Autodesk Inventor part; units mm, degrees
ref_plane "YZ Plane" through (0, 0, 0) normal (1, 0, 0) x (0, 1, 0)
ref_plane "XZ Plane" through (0, 0, 0) normal (0, 1, 0) x (-1, 0, 0)
ref_plane "XY Plane" through (0, 0, 0) normal (0, 0, 1) x (1, 0, 0)
sketch "Skizze1" plane through (0, 0, 0) normal (0, 0, 1) x (1, 0, 0)
  line L0 (0, 0) -> (90.4, 0)
  line L1 (90.4, 0) -> (90.4, 80)
  line L2 (90.4, 80) -> (0, 80)
  line L3 (0, 80) -> (0, 0)
  line L4 (2.6, 69.1) -> (87.8, 69.1) construction
  line L5 (87.8, 69.1) -> (87.8, 10.9) construction
  circle A0 centre (2.6, 69.1) radius 1.6
  circle A1 centre (2.6, 10.9) radius 1.6
  circle A2 centre (87.8, 69.1) radius 1.6
  circle A3 centre (87.8, 10.9) radius 1.6
  line L6 (65.2, 69.1) -> (82.75, 69.1) construction
  line L7 (25.2, 69.1) -> (42.75, 69.1) construction
  dimension "d0" = 90.4
  dimension "d1" = 80
  dimension "d5" = 87.8
  dimension "d6" = 3.2
extrude "Extrusion1" add sketch "Skizze1" along normal blind 2
chamfer "Fase1" distance 1.6 angle 45 4 edges at (86.2, 10.9, 2) (1, 10.9, 2) (1, 69.1, 2) (86.2, 69.1, 2)
properties part number "blech_2mm"
The model under review builds one solid part; all positions refer to its coordinate system, in mm. Coordinates: 2 decimals unless noted, no trailing zeros. Write each loop counter-clockwise with the first axis right and the second up, starting at its lowest first coordinate (ties: lowest second). Pieces come first, ordered by that corner, then holes. Notation, with made-up numbers: (59.25, -26) - (102.25, -26) arc R9 cw to (102.25, -11) - close; hole circle Ø4 at (17, -18.5). An arc over 180 degrees is marked (long way). Answer in a Markdown table with one row per item. Add a question column.
Q1. To check wall thickness, follow line 1 along Y through (x, z) = (87.8, 0.1); line 2 along X through (y, z) = (69.1, 0.2); line 3 along X through (y, z) = (11.5, 0.2). State the ranges of each line that lie inside material, in increasing order. Write a range as from..to.
Q2. Clearance check with flat-ended pins moving along their axes: pin 1 (4 mm diameter, centred on x = 87.8, y = 10.9, fed in from +Z); pin 2 (3 mm diameter, centred on x = 87.8, y = 69.1, fed in from +Z); pin 3 (5 mm diameter, centred on x = 2.6, y = 69.1, fed in from +Z). State where each tip first meets the part, or that it passes through.
Q3. Consider section A-A on x = 87.8. Give the boundary of the cut face in (y, z).
Q4. Consider section B-B on y = 10.9. Give the boundary of the cut face in (x, z).
Q5. Draft analysis for pull direction X (two halves, no side actions). For faces 1 (the face through (4.335, 10.181, 0.678)), 2 (the face through (45, 0, 1)), 3 (the face through (0, 41, 1)), state which applies: +X half, -X half, draft (parallel to the pull), parting line (faces both ways), or undercut.
Answers below:
| question | item | result |
|---|---|---|
| 1 | line 1 | 0..9.3, 12.5..67.5, 70.7..80 |
| 1 | line 2 | 0..1, 4.2..86.2, 89.4..90.4 |
| 1 | line 3 | 0..1.12, 4.08..86.32, 89.28..90.4 |
| 2 | pin 1 | z = 0.8 |
| 2 | pin 2 | through |
| 2 | pin 3 | z = 1.3 |
| 3 | outline | (0, 0) - (9.3, 0) - (9.3, 0.4) - (7.7, 2) - (0, 2) - close; (12.5, 0) - (67.5, 0) - (67.5, 0.4) - (65.9, 2) - (14.1, 2) - (12.5, 0.4) - close; (70.7, 0) - (80, 0) - (80, 2) - (72.3, 2) - (70.7, 0.4) - close |
| 4 | outline | (0, 0) - (1, 0) - (1, 0.4) - (0, 1.4) - close; (4.2, 0) - (86.2, 0) - (86.2, 0.4) - (84.6, 2) - (5.8, 2) - (4.2, 0.4) - close; (89.4, 0) - (90.4, 0) - (90.4, 1.4) - (89.4, 0.4) - close |
| 5 | face 1 | undercut |
| 5 | face 2 | draft |
| 5 | face 3 | -X half |
